```python
from build123d import *

# Parameters (mm, degrees)
SKETCH1_W           = 101.6
SKETCH1_H           = 50.8
BOSS_EXTRUDE1_DEPTH = 5.08
SKETCH2_R           = 8.382
BOSS_EXTRUDE2_DEPTH = 8.89
SKETCH4_W           = 101.6
SKETCH4_H           = 1.27
CUT_EXTRUDE1_DEPTH  = 1.27
SKETCH5_W           = 101.6
SKETCH5_H           = 1.27
CUT_EXTRUDE2_DEPTH  = 1.27


with BuildPart() as part:
    # Sketch1 → Boss-Extrude1 (new body)
    with BuildSketch(Plane(origin=(0, 0, 0), x_dir=(1, 0, 0), z_dir=(0, 1, 0))):
        with Locations((50.8, 25.4)):
            Rectangle(SKETCH1_W, SKETCH1_H)
    extrude(amount=BOSS_EXTRUDE1_DEPTH)

    # Sketch2 → Boss-Extrude2 (add)
    with BuildSketch(Plane(origin=(0, 0, 0), x_dir=(1, 0, 0), z_dir=(0, 1, 0))):
        with Locations(Location((50.8, 25.4, 0), (0, 0, 90))):
            Circle(SKETCH2_R)
    extrude(amount=BOSS_EXTRUDE2_DEPTH)

    # Sketch4 → Cut-Extrude1 (cut)
    with BuildSketch(Plane(origin=(0, 5.08, 0), x_dir=(1, 0, 0), z_dir=(0, 1, 0))):
        with Locations((50.8, 34.417)):
            Rectangle(SKETCH4_W, SKETCH4_H)
    extrude(amount=-CUT_EXTRUDE1_DEPTH, mode=Mode.SUBTRACT)

    # Sketch5 → Cut-Extrude2 (cut)
    with BuildSketch(Plane(origin=(0, 5.08, 0), x_dir=(1, 0, 0), z_dir=(0, 1, 0))):
        with Locations((50.8, 16.256)):
            Rectangle(SKETCH5_W, SKETCH5_H)
    extrude(amount=-CUT_EXTRUDE2_DEPTH, mode=Mode.SUBTRACT)


solid = part.part
```
CAD build for the part. Positions are in the model's coordinates, mm. A direction names the side the tool comes from. Round coordinates to 2 decimals unless told otherwise and drop trailing zeros. Write each loop counter-clockwise with the first axis right and the second up, starting at its lowest first coordinate (ties: lowest second). Pieces come first, ordered by that corner, then holes. Notation, with made-up numbers: (31.5, -20) - (85.5, -20) arc R5 cw to (85.5, -11) - close; hole circle Ø3 at (-33.5, 75). An arc over 180 degrees is marked (long way). Write item = value, one per line. Start each with the question number.
Q1. Which spindle directions (+Z, -Z, +X, -X, +Y, -Y) get a long thin tool onto all of the face, cutting with end or side? Do faces 1 (the flat face through (0, 3, -25)), 2 (the cylindrical face through (42.49, 6.96, -24.31)). Say none if no direction does.
Q2. Band-saw the part on B-B (x = 81). Give the cut face in (y, z).
Q3. Probe L1, parallel to Z at x = 91.5, y = 5; L2, parallel to Y at x = 39.5, z = -47; L3, parallel to Y at x = 58, z = -35. List the from-to ranges inside material, lowest first. Write a range as from..to.
Q4. Band-saw the part on A-A (z = -25.4). Give the cut face in (x, y), then the cut area to 3 significant figures.
Q5. Band-saw the part on C-C (y = 6.5). Give the cut face in (x, z), then the cut area to 3 significant figures.
Q6. Drop flat-ended pins along their axis: pin 1 (4 mm diameter, centred on x = 83, z = -16, fed in from +Y); pin 2 (1 mm diameter, centred on y = 7, z = -12, fed in from +X). Give the stop position or say it passes through.
Q7. Band-saw the part on D-D (z = -20). Give the cut face in (x, y).
Answers below:
q1.face_1 = +Z, -Z, -X, +Y, -Y
q1.face_2 = +Y
q2.outline = (0, -50.8) - (5.08, -50.8) - (5.08, -35.05) - (3.81, -35.05) - (3.81, -33.78) - (5.08, -33.78) - (5.08, -16.89) - (3.81, -16.89) - (3.81, -15.62) - (5.08, -15.62) - (5.08, 0) - (0, 0) - close
q3.L1 = -50.8..-35.05, -33.78..-16.89, -15.62..0
q3.L2 = 0..5.08
q3.L3 = 0..3.81
q4.outline = (0, 0) - (101.6, 0) - (101.6, 5.08) - (59.18, 5.08) - (59.18, 8.89) - (42.42, 8.89) - (42.42, 5.08) - (0, 5.08) - close
q4.area = 580 mm2
q5.outline = circle Ø16.76 at (50.8, -25.4)
q5.area = 221 mm2
q6.pin_1 = 5.08
q6.pin_2 = through
q7.outline = (0, 0) - (101.6, 0) - (101.6, 5.08) - (57.21, 5.08) - (57.21, 8.89) - (44.39, 8.89) - (44.39, 5.08) - (0, 5.08) - close
